Source: CAD feature listing. Evaluate the final solid. Frame: model axes, mm. A direction names the side the tool comes from. Give positions to 0.01 mm unless a question says otherwise; leave off trailing zeros. Order: outer loops, then holes, each group sorted by start corner. A loop starts at its lowest first (then second) coordinate and runs counter-clockwise, first axis right, second up. Notation, with made-up numbers: M -3,64.5 L 8,64.5 A19 cw 8,97.5 Z; hole C 39,19.25 d1. An arc over 180 degrees is marked long. Answer in a Markdown table with one row per item. Add a question column.
(1) Section query A-A, the plane y = -26.75. Return loops of the section in (x, z).
(2) Pin query (flat end, axial travel): P1, Ø4, axis at y = -32.5, z = -1.5, coming from the +X side. Return the tip coordinate at first contact, or that it passes through.
(3) Section query C-C, the plane z = 0. Return loops of the section in (x, y), plus the area to 3 significant figures.
(4) Section query B-B, the plane y = -41.5. Return loops of the section in (x, z).
(5) Material intervals for line 1 along Y through (x, z) = (-8.5, -1.75); line 2 along Y through (x, z) = (-11, 0.75); line 3 along Z through (x, y) = (-11, -25.75), sorted ascending.
(6) Set-up query: faces 1 (the face through (-6.316, -27.175, 0.159)), 2 (the face through (-8.77, -25.99, -1.02)), 3 (the face through (-11.77, -36.74, -0.77)). Return all of +Z, -Z, +X, -X, +Y, -Y with unobstructed straight access to the full face (end or side cutting, diameter ignored); none if empty.
Autodesk Inventor part; units mm, degrees
ref_plane "YZ Plane" through (0, 0, 0) normal (1, 0, 0) x (0, 1, 0)
ref_plane "XZ Plane" through (0, 0, 0) normal (0, 1, 0) x (-1, 0, 0)
ref_plane "XY Plane" through (0, 0, 0) normal (0, 0, 1) x (1, 0, 0)
sketch "Sketch1" plane through (0, 0, 0) normal (0, 0, 1) x (1, 0, 0)
  line L0 (-9.9228, -29) -> (-13.5328, -29)
  line L1 (-13.5328, -29) -> (-13.5328, -25)
  line L2 (-13.5328, -25) -> (-9.9228, -25)
  line L3 (-9.9228, -25) -> (-9.9228, -29)
  line L4 (-9.9228, -29) -> (-9.9228, -45)
  line L5 (-9.9228, -45) -> (-11.9228, -45)
  line L6 (-11.9228, -45) -> (-11.9228, -29)
  point P0 (0, 0)
  dimension "d0" = 3.61
  dimension "d1" = 4
  dimension "d2" = 16
  dimension "d3" = 2
revolve "Revolution1" add sketch "Sketch1" angle 360 about axis through (-9.9228, -29, 0) along (0, -1, 0)
chamfer "Chamfer1" distance 0.4 angle 45 1 edges at (-6.3128, -25, 0)
sketch "Boceto2" plane through (-9.9228, -25, 0) normal (0, 1, 0) x (1, 0, 0)
  line L0 (1.1641, -1.3443) -> (-0.5821, -1.6803)
  line L1 (-0.5821, -1.6803) -> (-1.7462, -0.336)
  line L2 (-1.7462, -0.336) -> (-1.1641, 1.3443)
  line L3 (-1.1641, 1.3443) -> (0.5821, 1.6803)
  line L4 (0.5821, 1.6803) -> (1.7462, 0.336)
  line L5 (1.7462, 0.336) -> (1.1641, -1.3443)
  point P0 (9.9228, 0)
  point P1 (0, 0)
  dimension "d11" = 3.08
extrude "Extrusión1" cut sketch "Boceto2" against normal blind 2
thread "Rosca1"
chamfer "Chamfer3" distance 0.3 angle 45 1 edges at (-7.9228, -45, 0)
properties part number "Tornillo Allen cabeza cilindrica M4x16mm"
Values follow:
| question | item | result |
|---|---|---|
| 1 | outline | C -9.92,0 d7.22; hole M -11.67,0.34 L -11.09,-1.34 L -9.34,-1.68 L -8.18,-0.34 L -8.76,1.34 L -10.5,1.68 Z |
| 2 | P1 | stops at x = -7.92 |
| 3 | outline | M -13.53,-29 L -11.92,-29 L -11.92,-44.7 L -11.62,-45 L -8.22,-45 L -7.92,-44.7 L -7.92,-29 L -6.31,-29 L -6.31,-25.4 L -6.71,-25 L -8.29,-25 L -8.29,-27 L -11.55,-27 L -11.55,-25 L -13.13,-25 L -13.53,-25.4 Z |
| 3 | area | 86.1 mm² |
| 4 | outline | C -9.92,0 d4 |
| 5 | line 1 | y = -29 to -25 |
| 5 | line 2 | y = -45 to -27 |
| 5 | line 3 | z = -3.45 to -1.36, 1.11 to 3.45 |
| 6 | face 1 | +Y, -Y |
| 6 | face 2 | +Y |
| 6 | face 3 | -Y |
